The model under review builds one solid part; all positions refer to its coordinate system, in mm. Face numbers are marked on the shaded views. Give positions to 0.01 mm unless a question says otherwise; leave off trailing zeros. Order: outer loops, then holes, each group sorted by start corner. A loop starts at its lowest first (then second) coordinate and runs counter-clockwise, first axis right, second up. Notation, with made-up numbers: M 42,-8 L 77,-8 A24 cw 77,25 Z; hole C -4,-26.5 d3. An arc over 180 degrees is marked long. One line per question, with ' | ' between items. Start each with the question number.
1. The part is to be moulded in two halves that separate along X. For the marked faces 1 and 2, say which applies: +X half, -X half, draft (parallel to the pull), parting line (faces both ways), or undercut.
2. Insertion check: P1, Ø3.5, axis at x = 34.97, y = -35.02, coming from the +Z side; P2, Ø20, axis at x = 9, y = 9.5, coming from the -Z side. Each pin has a flat end and moves straight along its axis. Give the tip position at first contact, or say it passes through.
3. Wall thickness on L1, parallel to Y at x = 20, z = 3.5; L2, parallel to X at y = -34, z = 1.8: over which ranges is each line inside the solid? List them lowest first.
4. We need section D-D on z = 3.1. Count the separate pieces of the cut face and the enclosed holes in it, then the cut area to 3 significant figures.
5. We need section A-A on y = 0. Write out the cut boundary in (x, z).
6. We need section C-C on x = -18. Write out the cut boundary in (y, z), then the cut area to 3 significant figures.
```python
from build123d import *

# Parameters (mm, degrees)
BOSS_EXTRU_1_DEPTH      = 5
D_GAGEMENT_M41_D        = 4.5
ESQUISSE4_R             = 3.25
ENL_V_MAT_EXTRU_1_DEPTH = 57.789083458
D_GAGEMENT_M61_D        = 6.6
ENL_V_MAT_EXTRU_2_DEPTH = 2


with BuildPart() as part:
    # Esquisse1 → Boss.-Extru.1 (new body)
    with BuildSketch(Plane.XY):
        with BuildLine():
            Line((-36, -40), (36, -40))
            ThreePointArc((36, -40), (38.828427125, -38.828427125), (40, -36))
            Line((40, -36), (40, 36))
            ThreePointArc((40, 36), (38.828427125, 38.828427125), (36, 40))
            Line((36, 40), (-36, 40))
            ThreePointArc((-36, 40), (-38.828427125, 38.828427125), (-40, 36))
            Line((-40, 36), (-40, -36))
            ThreePointArc((-40, -36), (-38.828427125, -38.828427125), (-36, -40))
        make_face()
    extrude(amount=BOSS_EXTRU_1_DEPTH)

    # Dégagement M41 (through all)
    with Locations(Plane.XY.offset(5)):
        with Locations((-35.007622699, 34.962380164), (34.968353645, 34.962380164), (34.968353645, -35.023881333), (-35.007622699, -35.023881333)):
            Hole(D_GAGEMENT_M41_D / 2)

    # Esquisse4 → Enlèv. mat.-Extru.1 (cut, through all)
    with BuildSketch(Plane(origin=(0, 0, 0), x_dir=(-1, 0, 0), z_dir=(0, 0, -1))):
        Circle(ESQUISSE4_R)
    extrude(amount=-ENL_V_MAT_EXTRU_1_DEPTH, mode=Mode.SUBTRACT)

    # Dégagement M61 (through all)
    with Locations(Plane.XY.offset(5)):
        with Locations((-20, 20), (20, 20), (20, -20), (-20, -20)):
            Hole(D_GAGEMENT_M61_D / 2)

    # Esquisse7 → Enlèv. mat.-Extru.2 (cut)
    with BuildSketch(Plane(origin=(0, 0, 0), x_dir=(-1, 0, 0), z_dir=(0, 0, -1))):
        with BuildLine():
            Line((-16, 20), (16, 20))
            add(Edge.make_bspline(
                [(16, 20), (19.65685425, 19.656854249), (20, 16)],
                knots=[0, 0, 0, 1, 1, 1], degree=2))
            Line((20, 16), (20, -16))
            add(Edge.make_bspline(
                [(20, -16), (19.65685425, -19.65685425), (16, -20)],
                knots=[0, 0, 0, 1, 1, 1], degree=2))
            Line((16, -20), (-16, -20))
            add(Edge.make_bspline(
                [(-16, -20), (-19.656854249, -19.65685425), (-20, -16)],
                knots=[0, 0, 0, 1, 1, 1], degree=2))
            Line((-20, -16), (-20, 16))
            add(Edge.make_bspline(
                [(-20, 16), (-19.656854249, 19.656854249), (-16, 20)],
                knots=[0, 0, 0, 1, 1, 1], degree=2))
        make_face()
    extrude(amount=-ENL_V_MAT_EXTRU_2_DEPTH, mode=Mode.SUBTRACT)


solid = part.part
```
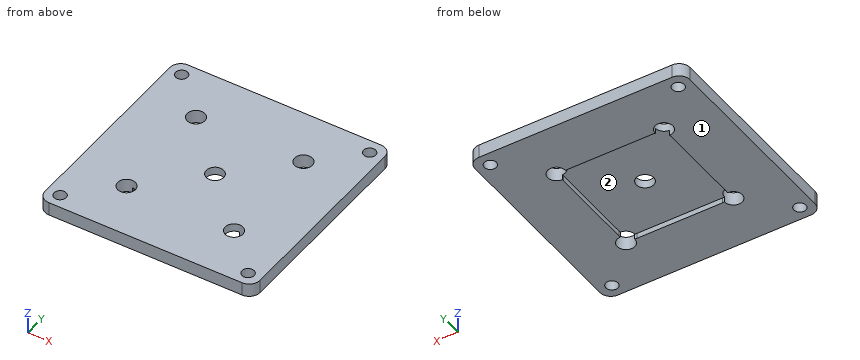
Entries:
1) face 1: draft | face 2: undercut
2) P1: passes through | P2: stops at z = 2
3) L1: y = -40 to -23.3, -16.7 to 16.7, 23.3 to 40 | L2: x = -40 to -37.01, -33 to 32.96, 36.97 to 40
4) separate pieces: 1 | enclosed holes: 9 | area: 6,150 mm^2
5) outline: M -40,0 L -20,0 L -20,2 L -3.25,2 L -3.25,5 L -40,5 Z; M 3.25,2 L 20,2 L 20,0 L 40,0 L 40,5 L 3.25,5 Z
6) outline: M -40,0 L -22.62,0 L -22.62,5 L -40,5 Z; M -17.38,2 L 17.38,2 L 17.38,5 L -17.38,5 Z; M 22.62,0 L 40,0 L 40,5 L 22.62,5 Z | area: 278 mm^2
